from build123d import *

# Parameters (mm, degrees)
F0_R     = 1.190625
F0_R_2   = 1.5875
F1_DEPTH = 1.5875


with BuildPart() as f1:
    # F0 (on Front) → F1 (new body, symmetric)
    with BuildSketch(Plane.XZ):
        with BuildLine():
            Line((-4.19507, -3.443071), (-4.164685, -4.719849))
            ThreePointArc((-4.164685, -4.719849), (6.575626, 10.980695), (-5.78257, -3.480852))
            Line((-5.78257, -3.480852), (-4.19507, -3.443071))
        make_face()
        with Locations((7.395771, 0.439879)):
            Circle(F0_R, mode=Mode.SUBTRACT)
        with Locations((0.784385, 3.418477)):
            Circle(F0_R_2, mode=Mode.SUBTRACT)
    extrude(amount=F1_DEPTH, both=True)


solid = f1.part
Verification items for the finished model (mm, model axes). Coordinates: 2 decimals unless noted, no trailing zeros. Order: outer loops, then holes, each group sorted by start corner. A loop starts at its lowest first (then second) coordinate and runs counter-clockwise, first axis right, second up.
1. Release check for a two-part mould opening along Z. For faces 1 (the face through (6.89, -0.02, 10.73)), 2 (the face through (1, 1.588, 1)), 3 (the face through (6.206, 0.022, 0.492)) record: +Z half, -Z half, draft (parallel to the pull), parting line (faces both ways), or undercut.
Results found:
face 1: parting line
face 2: draft
face 3: undercut
2. Sectioned sample at D-D, the plane z = 7. Record the cut outline in (x, y), and give its area (3 significant figures).
Results found:
outline: (-8.04, -1.59) - (9.61, -1.59) - (9.61, 1.59) - (-8.04, 1.59) - close
area: 56.0 mm2
3. Sectioned sample at B-B, the plane z = 2.5. Record the cut outline in (x, y) (1 decimal).
Results found:
outline: (-8.7, -1.6) - (-0.5, -1.6) - (-0.5, 1.6) - (-8.7, 1.6) - close; (2.1, -1.6) - (10.3, -1.6) - (10.3, 1.6) - (2.1, 1.6) - close
4. Sectioned sample at A-A, the plane x = 0.25. Record the cut outline in (y, z).
Results found:
outline: (-1.59, -6.09) - (1.59, -6.09) - (1.59, 1.92) - (-1.59, 1.92) - close; (-1.59, 4.91) - (1.59, 4.91) - (1.59, 12.93) - (-1.59, 12.93) - close
5. Scan lines: line 1 (X direction, y = 1.4, z = 3); line 2 (X direction, y = -0.95, z = 4.5); line 3 (Z direction, x = 7.75, y = 1.1). Record each from-to range of solid material in increasing order.
Results found:
line 1: x = -8.73 to -0.75, 2.32 to 10.3
line 2: x = -8.68 to -0.38, 1.95 to 10.25
line 3: z = -3.08 to -0.7, 1.58 to 9.92
6. Go/stop test with flat-tipped pins: pin 1 Ø1 at (y, z) = (1, -4) entering from +X; pin 2 Ø1 at (x, y) = (8, 0) entering from +Z. Record where each tip stops, or that it passes through.
Results found:
pin 1: stops at x = 7.33
pin 2: stops at z = 10.17
7. Sectioned sample at C-C, the plane y = -0.15. Give the number of separate pieces and of enclosed holes in the cut face, and give its area (3 significant figures).
Results found:
separate pieces: 1
enclosed holes: 2
area: 272 mm2
